Source: three-view drawing plus pictorial views. Frame: mm from the lowest corner of the part. A direction names the side the tool comes from. Round coordinates to 2 decimals unless told otherwise and drop trailing zeros. Order: outer loops, then holes, each group sorted by start corner. A loop starts at its lowest first (then second) coordinate and runs counter-clockwise, first axis right, second up. Notation, with made-up numbers: M -28,14.25 L -3,14.25 A19 ccw -3,20.25 Z; hole C -18,53 d1. An arc over 180 degrees is marked long. Return JSON: item names as keys, results as strings. Group by question number.
Q1. Cut plane C-C on x = 10. Output: boundary loops of the cut face in (y, z).
Q2. Ray query, probe 1 along Y at (x, z) = (10, 19.3); probe 2 along Y at (x, z) = (10, 19.5); probe 3 along X at (y, z) = (0.4, 15). Return the intervals inside material, ascending.
Q3. Cut plane A-A on z = 15. Output: boundary loops of the cut face in (x, y).
Q4. Contact query for flat-ended pins moving along their axis: pin 1 (1.5 mm diameter, centred on x = 13.5, y = 11, fed in from -Z); pin 2 (6.5 mm diameter, centred on x = 10, z = 7, fed in from +Y). Output: stop coordinate, or through.
Q5. Cut plane D-D on x = 14.5. Output: boundary loops of the cut face in (y, z), and give its area (3 significant figures).
Q6. Cut plane B-B on y = 7. Output: boundary loops of the cut face in (x, z), and give its area (3 significant figures).
Q7. Access query for the marked faces 1 and 2. Directions: +Z, -Z, +X, -X, +Y, -Y. A direction counts if a zero-diameter tool reaches every point of the face in a straight line with its end or side. Return the directions, or none.
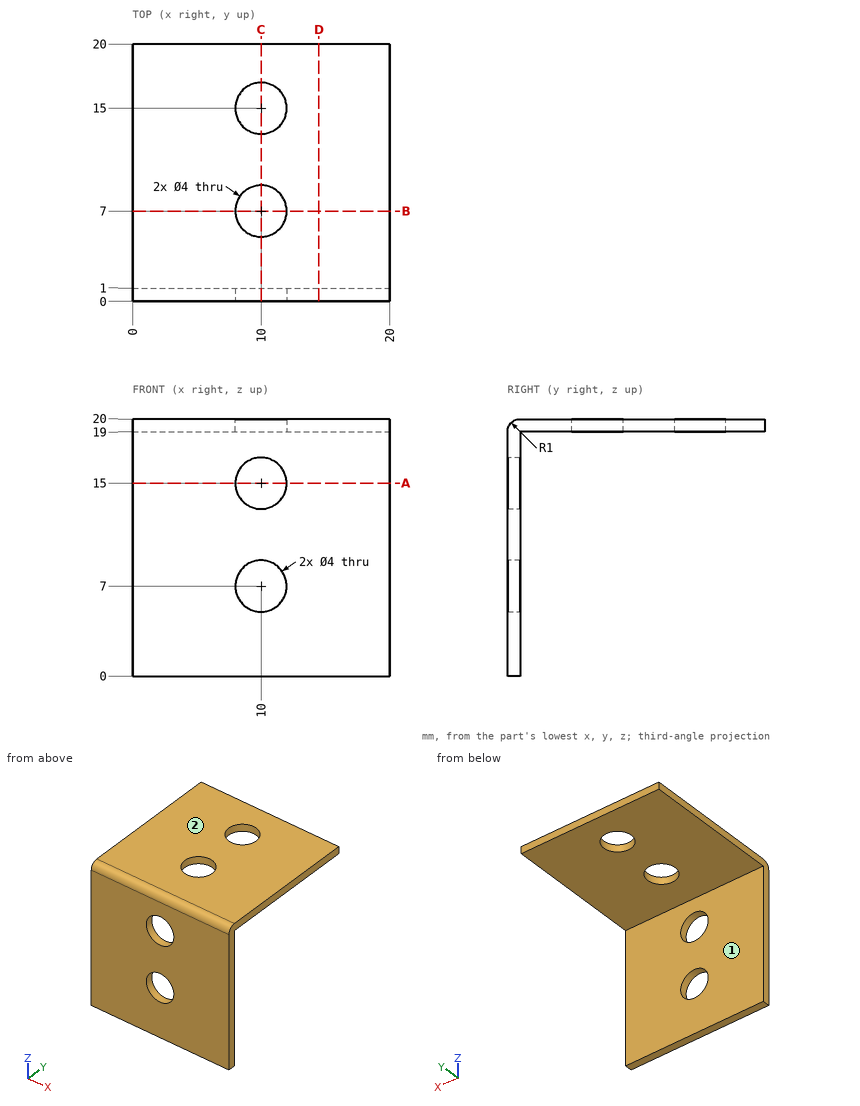
Result sheet:
{
 "1": {"outline": "M 0,0 L 1,0 L 1,5 L 0,5 Z; M 0,9 L 1,9 L 1,13 L 0,13 Z; M 0,17 L 1,17 L 1,19 L 5,19 L 5,20 L 1,20 A1 ccw 0,19 Z; M 9,19 L 13,19 L 13,20 L 9,20 Z; M 17,19 L 20,19 L 20,20 L 17,20 Z"},
 "2": {"probe 1": "y = 0.05 to 5, 9 to 13, 17 to 20", "probe 2": "y = 0.13 to 5, 9 to 13, 17 to 20", "probe 3": "x = 0 to 8, 12 to 20"},
 "3": {"outline": "M 0,0 L 8,0 L 8,1 L 0,1 Z; M 12,0 L 20,0 L 20,1 L 12,1 Z"},
 "4": {"pin 1": "stops at z = 19", "pin 2": "stops at y = 1"},
 "5": {"outline": "M 0,0 L 1,0 L 1,19 L 20,19 L 20,20 L 1,20 A1 ccw 0,19 Z", "area": "38.8 mm²"},
 "6": {"outline": "M 0,19 L 8,19 L 8,20 L 0,20 Z; M 12,19 L 20,19 L 20,20 L 12,20 Z", "area": "16.0 mm²"},
 "7": {"face 1": "-Z, +X, -X, +Y", "face 2": "+Z, +X, -X, +Y, -Y"}
}
